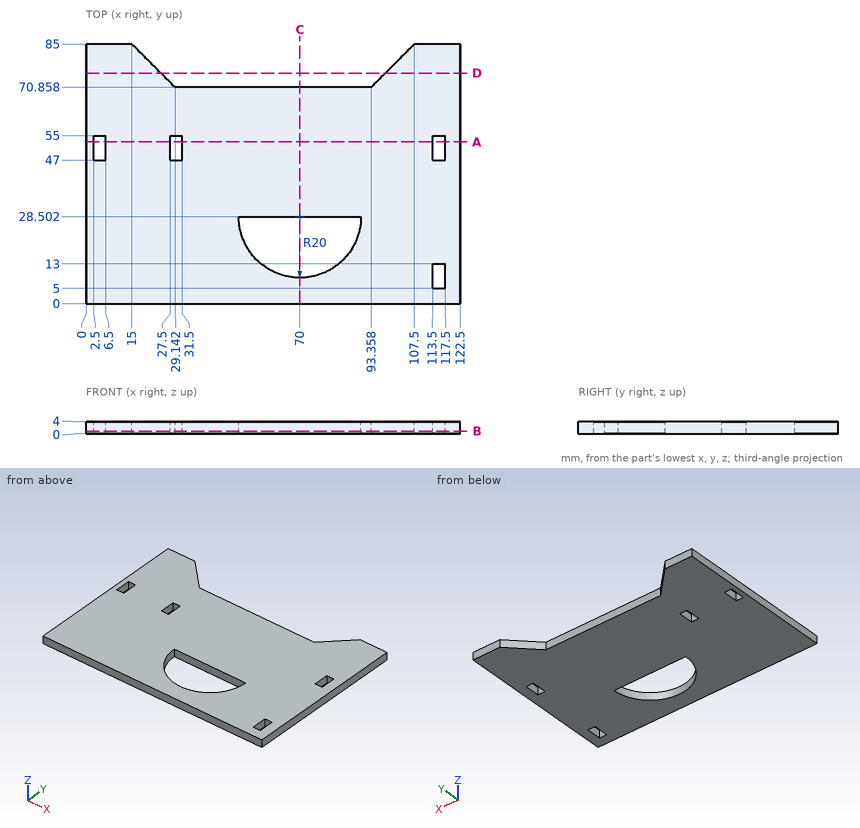
Part print with two shaded views. Sizes in mm from the minimum x, y, z corner. Round coordinates to 2 decimals unless told otherwise and drop trailing zeros. Write each loop counter-clockwise with the first axis right and the second up, starting at its lowest first coordinate (ties: lowest second). Pieces come first, ordered by that corner, then holes. Notation, with made-up numbers: M 13,-7.5 L 19,-7.5 A30 ccw 19,26.5 Z; hole C 74.5,28 d11. An arc over 180 degrees is marked long. Put each result on its own line as item: value. Start each with the question number.
1) Drill centre lines: probe 1 along X at (y, z) = (51, 3.2); probe 2 along Y at (x, z) = (114.5, 2.45); probe 3 along Y at (x, z) = (69.5, 2.6). Where is each one in solid material? Low to high. Write a range as [from, to].
2) Saw through at D-D, the plane y = 75.5. Write the cut outline in (x, z), and give its area (3 significant figures).
3) Saw through at B-B, the plane z = 0.9. Write the cut outline in (x, y).
4) Pin check, flat tips, straight feed: pin 1 Ø2 at (x, z) = (30.5, 1) entering from +Y; pin 2 Ø2 at (y, z) = (51, 2) entering from -X. Stop position of each tip, or through.
5) Saw through at C-C, the plane x = 70. Write the cut outline in (y, z).
6) Saw through at A-A, the plane y = 53. Write the cut outline in (x, z), and give its area (3 significant figures).
Resolved:
1. probe 1: [0, 2.5], [6.5, 27.5], [31.5, 113.5], [117.5, 122.5]
1. probe 2: [0, 5], [13, 47], [55, 85]
1. probe 3: [0, 8.51], [28.5, 70.86]
2. outline: M 0,0 L 24.5,0 L 24.5,4 L 0,4 Z; M 98,0 L 122.5,0 L 122.5,4 L 98,4 Z
2. area: 196 mm²
3. outline: M 0,0 L 122.5,0 L 122.5,85 L 107.5,85 L 93.36,70.86 L 29.14,70.86 L 15,85 L 0,85 Z; hole M 2.5,47 L 6.5,47 L 6.5,55 L 2.5,55 Z; hole M 27.5,47 L 31.5,47 L 31.5,55 L 27.5,55 Z; hole M 50,28.5 A20 ccw 90,28.5 Z; hole M 113.5,5 L 117.5,5 L 117.5,13 L 113.5,13 Z; hole M 113.5,47 L 117.5,47 L 117.5,55 L 113.5,55 Z
4. pin 1: y = 70.86
4. pin 2: x = 0
5. outline: M 0,0 L 8.5,0 L 8.5,4 L 0,4 Z; M 28.5,0 L 70.86,0 L 70.86,4 L 28.5,4 Z
6. outline: M 0,0 L 2.5,0 L 2.5,4 L 0,4 Z; M 6.5,0 L 27.5,0 L 27.5,4 L 6.5,4 Z; M 31.5,0 L 113.5,0 L 113.5,4 L 31.5,4 Z; M 117.5,0 L 122.5,0 L 122.5,4 L 117.5,4 Z
6. area: 442 mm²
